Check sheet for the drawn part. Datum: minimum x, y, z corner. Units: mm. Coordinates: 2 decimals unless noted, no trailing zeros. Order: outer loops, then holes, each group sorted by start corner. A loop starts at its lowest first (then second) coordinate and runs counter-clockwise, first axis right, second up. Notation, with made-up numbers: M 44.25,18.25 L 59.25,18.25 A15 cw 59.25,25.25 Z; hole C 0,-14 d7. An arc over 180 degrees is marked long. Return JSON: item names as keys, results as strings. Group by question number.
Q1. Section check B-B, the plane z = 0.8. Count the separate pieces of the cut face and the enclosed holes in it, then the cut area to 3 significant figures.
Q2. Section check D-D, the plane x = 93.5. Enter the section's corners in (y, z).
Q3. Section check C-C, the plane y = 70.5. Enter the section's corners in (x, z).
Q4. Thickness scan on probe 1 along Y at (x, z) = (39.45, 1.2); probe 2 along Y at (x, z) = (33, 1.2); probe 3 along Y at (x, z) = (94.5, 2.7). Record the ranges inside material, lowest first.
Q5. Section check A-A, the plane x = 34.45. Enter the section's corners in (y, z).
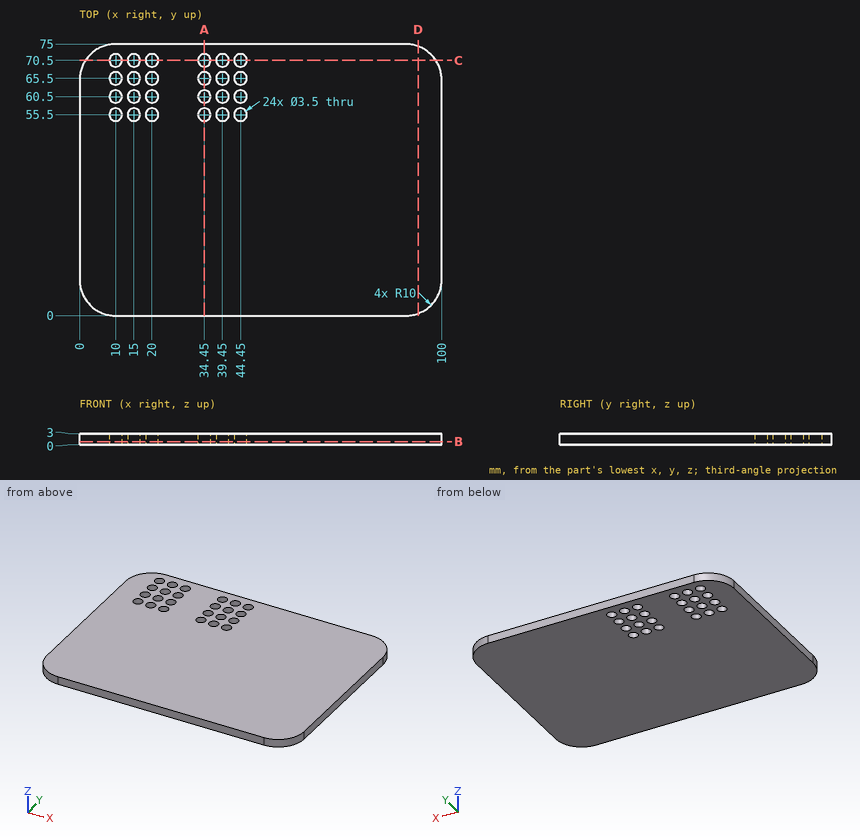
Numbers:
{
 "1": {"separate pieces": "1", "enclosed holes": "24", "area": "7,180 mm2"},
 "2": {"outline": "M 0.63,0 L 74.37,0 L 74.37,3 L 0.63,3 Z"},
 "3": {"outline": "M 1.65,0 L 8.25,0 L 8.25,3 L 1.65,3 Z; M 11.75,0 L 13.25,0 L 13.25,3 L 11.75,3 Z; M 16.75,0 L 18.25,0 L 18.25,3 L 16.75,3 Z; M 21.75,0 L 32.7,0 L 32.7,3 L 21.75,3 Z; M 36.2,0 L 37.7,0 L 37.7,3 L 36.2,3 Z; M 41.2,0 L 42.7,0 L 42.7,3 L 41.2,3 Z; M 46.2,0 L 98.35,0 L 98.35,3 L 46.2,3 Z"},
 "4": {"probe 1": "y = 0 to 53.75, 57.25 to 58.75, 62.25 to 63.75, 67.25 to 68.75, 72.25 to 75", "probe 2": "y = 0 to 54.52, 56.48 to 59.52, 61.48 to 64.52, 66.48 to 69.52, 71.48 to 75", "probe 3": "y = 1.07 to 73.93"},
 "5": {"outline": "M 0,0 L 53.75,0 L 53.75,3 L 0,3 Z; M 57.25,0 L 58.75,0 L 58.75,3 L 57.25,3 Z; M 62.25,0 L 63.75,0 L 63.75,3 L 62.25,3 Z; M 67.25,0 L 68.75,0 L 68.75,3 L 67.25,3 Z; M 72.25,0 L 75,0 L 75,3 L 72.25,3 Z"}
}
